```python
from build123d import *

# Parameters (mm, degrees)
F0_R     = 12.7
F1_DEPTH = 635
F2_R     = 25.153949
F3_DEPTH = 20.32
F5_W     = 35.0695
F5_H     = 31.220594
F6_DEPTH = 2.54


with BuildPart() as f1:
    # F0 (on Top) → F1 (new body)
    with BuildSketch(Plane.XY):
        Circle(F0_R)
    extrude(amount=F1_DEPTH)

    # F2 (on Front) → F3 (join)
    with BuildSketch(Plane.XZ):
        with Locations((-12.71527, 0)):
            Circle(F2_R)
    extrude(amount=F3_DEPTH)

    # F4: F1 across plane


with BuildPart() as f1_1:
    add(f1.part)
    add(f1.part.mirror(Plane.XZ))

    # F5 (on face) → F6 (join)
    with BuildSketch(Plane.XY.offset(635)):
        Rectangle(F5_W, F5_H)
    extrude(amount=F6_DEPTH)


solid = f1_1.part
```
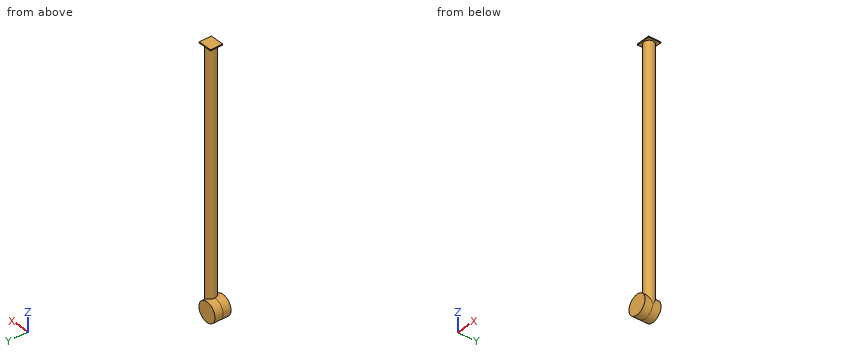
The model under review builds one solid part; all positions refer to its coordinate system, in mm. Round coordinates to 2 decimals unless told otherwise and drop trailing zeros. Loops run counter-clockwise (first coordinate to the right, second up) from the corner with the lowest first, then second, coordinate; pieces in that order, holes last.
1) Consider section B-B on z = 450. State the section outline as (x, y) points, then the cut area to 3 significant figures.
Values follow:
outline: circle Ø25.4 at (0, 0)
area: 507 mm2
2) Consider section C-C on x = -27. State the section outline as (y, z) points.
Values follow:
outline: (-20.32, -20.7) - (20.32, -20.7) - (20.32, 20.7) - (-20.32, 20.7) - close
3) Clearance check with flat-ended pins moving along their axes: P1, Ø3, axis at y = -7, z = 636.5, coming from the -X side; P2, Ø1, axis at x = -8.5, z = 496, coming from the +Y side; P3, Ø10, axis at x = -3, y = 4.5, coming from the -Z side. State where each tip first meets the part, or that it passes through.
Values follow:
P1: stops at x = -17.53
P2: stops at y = 9.86
P3: stops at z = -24.71
4) Consider section A-A on x = 0. State the section outline as (y, z) points.
Values follow:
outline: (-20.32, -21.7) - (20.32, -21.7) - (20.32, 21.7) - (12.7, 21.7) - (12.7, 635) - (15.61, 635) - (15.61, 637.54) - (-15.61, 637.54) - (-15.61, 635) - (-12.7, 635) - (-12.7, 21.7) - (-20.32, 21.7) - close
5) Wall thickness on line 1 along Y through (x, z) = (0.5, 491.5); line 2 along Z through (x, y) = (13.5, 10); line 3 along X through (y, z) = (-1, 230): over which ranges is each line inside the solid? List them lowest first.
Values follow:
line 1: y = -12.69 to 12.69
line 2: z = 635 to 637.54
line 3: x = -12.66 to 12.66
